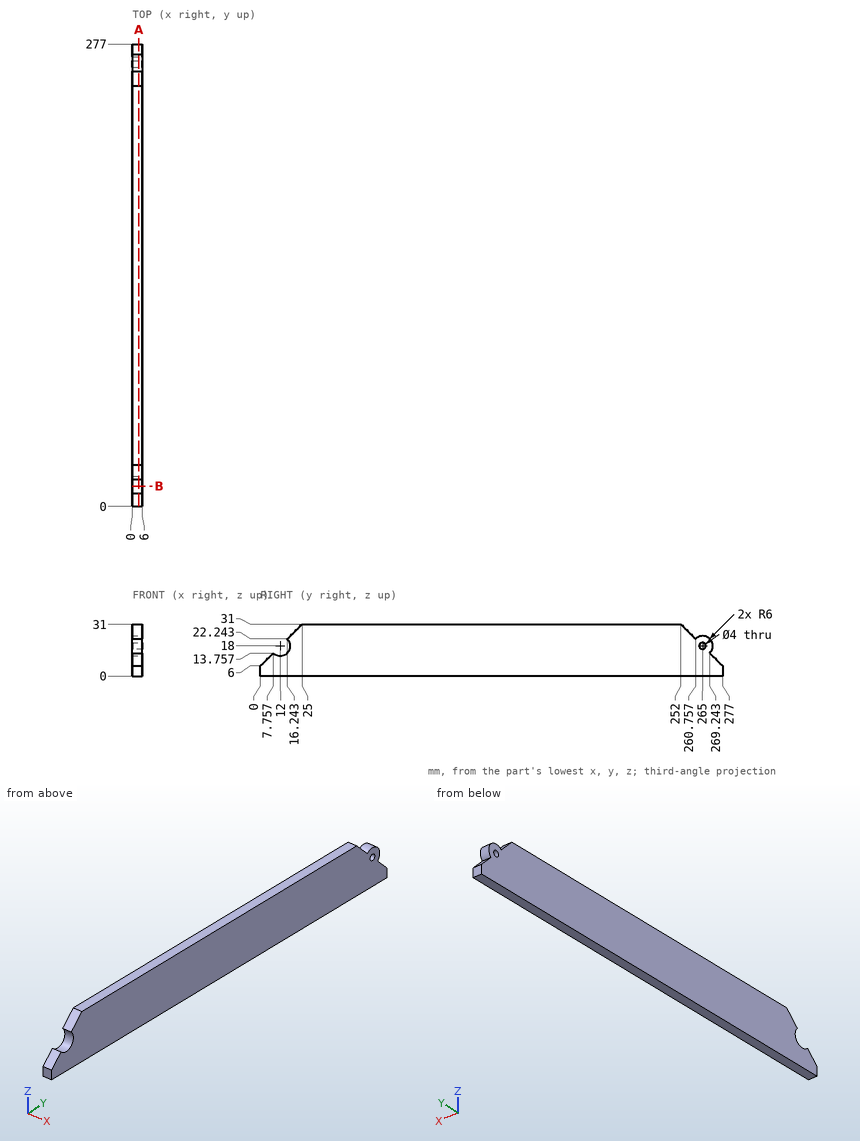
Could you check a few things on this drawing? It's one solid part, dimensions in mm from its lowest x, y, z. Round coordinates to 2 decimals unless told otherwise and drop trailing zeros. Order: outer loops, then holes, each group sorted by start corner. A loop starts at its lowest first (then second) coordinate and runs counter-clockwise, first axis right, second up. Notation, with made-up numbers: M -13.75,36.25 L -1.75,36.25 A34 cw -1.75,67.25 Z; hole C -14,29.5 d3. An arc over 180 degrees is marked long. One line per item, written item: value.
(1) Imagine slicing it at B-B (y = 12). Write out the boundary of the cut face in (x, z).
Ans:
outline: M 0,0 L 6,0 L 6,12 L 0,12 Z
(2) I'm going to push flat-ended pins straight in: P1, Ø3, axis at x = 2.5, z = 17, coming from the -Y side (1 decimal); P2, Ø2, axis at x = 4.5, y = 165.5, coming from the -Z side; P3, Ø1.5, axis at x = 3.5, z = 22.5, coming from the +Y side (1 decimal). Where does each tip first touch, or does it pass through?
Ans:
P1: stops at y = 17.5
P2: stops at z = 0
P3: stops at y = 269.7
(3) Imagine slicing it at A-A (x = 3.9). Write out the boundary of the cut face in (y, z).
Ans:
outline: M 0,0 L 277,0 L 277,6 L 269.24,13.76 A6 ccw 260.76,22.24 L 252,31 L 25,31 L 16.24,22.24 A6 cw 7.76,13.76 L 0,6 Z; hole C 265,18 d4
(4) I need wall thicknesses on line 1 along Y through (x, z) = (2.15, 18); line 2 along Z through (x, y) = (2.1, 265); line 3 along Y through (x, z) = (2, 23) (1 decimal). Which ranges of each line are inside material? Lowest first, please. Write a range as from..to.
Ans:
line 1: y = 18..263, 267..271
line 2: z = 0..16, 20..24
line 3: y = 17..260, 261.7..268.3
